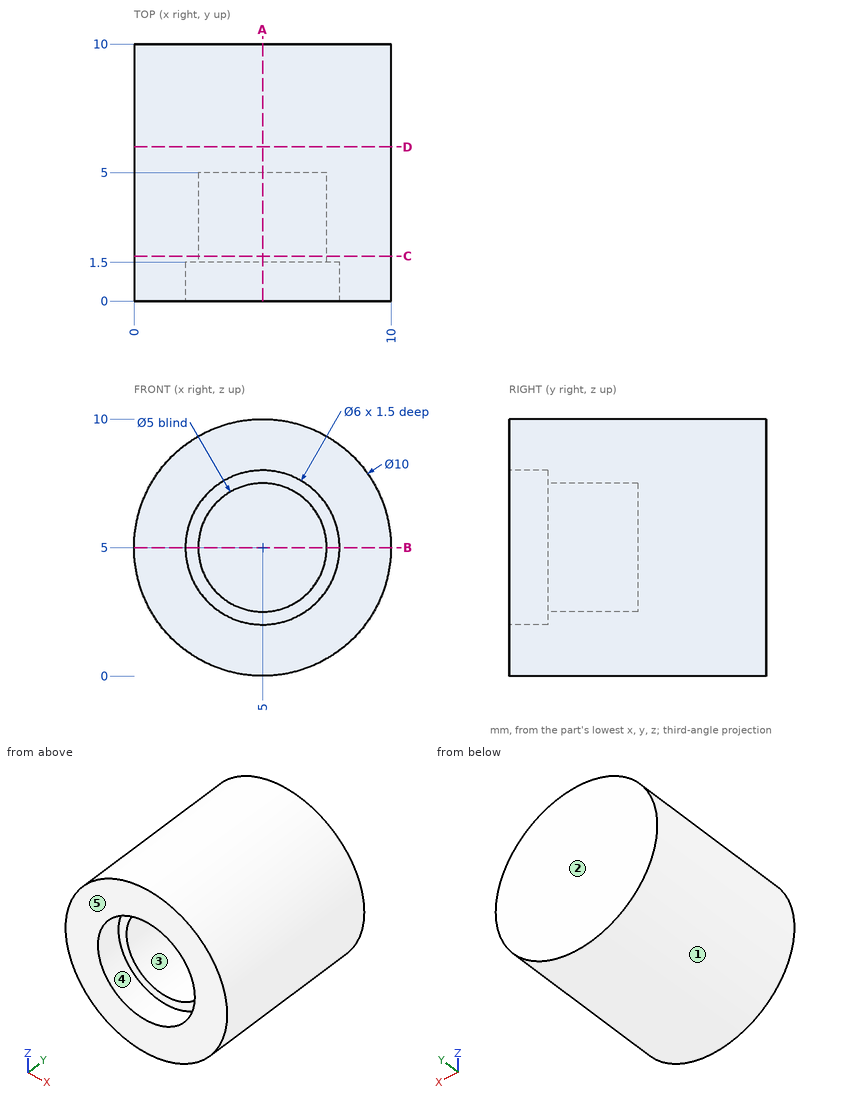
The figure shows three views and two pictorial views of one solid part (mm, origin at its lowest corner). Answer the questions. A direction names the side the tool comes from. Round coordinates to 2 decimals unless told otherwise and drop trailing zeros. Write each loop counter-clockwise with the first axis right and the second up, starting at its lowest first coordinate (ties: lowest second). Pieces come first, ordered by that corner, then holes. Notation, with made-up numbers: M -29.75,38.25 L 27.25,38.25 A29 ccw 27.25,76.25 Z; hole C -32,-15 d2. An arc over 180 degrees is marked long. Use a Markdown table: item, result.
1) The part is cut by section A-A (x = 5). Write down the section's boundary in (y, z).
Answers follow:
| item | result |
|---|---|
| outline | M 0,0 L 10,0 L 10,10 L 0,10 L 0,8 L 1.5,8 L 1.5,7.5 L 5,7.5 L 5,2.5 L 1.5,2.5 L 1.5,2 L 0,2 Z |
2) Straight lines are drawn through the part: line 1 along Z through (x, y) = (5, 2.95); line 2 along Y through (x, z) = (3.5, 6.5); line 3 along X through (y, z) = (4, 6.25). For each, find the intervals that lie inside material, in ascending order. Write a range as [from, to].
Answers follow:
| item | result |
|---|---|
| line 1 | z = [0, 2.5], [7.5, 10] |
| line 2 | y = [5, 10] |
| line 3 | x = [0.16, 2.83], [7.17, 9.84] |
3) The part is cut by section B-B (z = 5). Write down the section's boundary in (x, y).
Answers follow:
| item | result |
|---|---|
| outline | M 0,0 L 2,0 L 2,1.5 L 2.5,1.5 L 2.5,5 L 7.5,5 L 7.5,1.5 L 8,1.5 L 8,0 L 10,0 L 10,10 L 0,10 Z |
4) The part is cut by section C-C (y = 1.75). Write down the section's boundary in (x, z).
Answers follow:
| item | result |
|---|---|
| outline | C 5,5 d10; hole C 5,5 d5 |
5) Flat-ended cylindrical pins translate along their axes: pin 1 (4 mm diameter, centred on x = 2.5, y = 2, fed in from -Z); pin 2 (3 mm diameter, centred on x = 1.5, y = 5, fed in from +Z); pin 3 (1.5 mm diameter, centred on x = 1.5, y = 8.5, fed in from +Z). Find the tip coordinate at first contact, or state that the pin passes through.
Answers follow:
| item | result |
|---|---|
| pin 1 | stops at z = 0.03 |
| pin 2 | stops at z = 9.58 |
| pin 3 | stops at z = 9.18 |
6) For a pull along X with two mould halves and no side action, classify the marked faces 1, 2 and 3 as pulls with the +X half, pulls with the -X half, needs draft (parallel to the pull), parting line crosses it, or undercut.
Answers follow:
| item | result |
|---|---|
| face 1 | parting line crosses it |
| face 2 | needs draft |
| face 3 | undercut |
7) The part is cut by section D-D (y = 6). Write down the section's boundary in (x, z), plus the area to 3 significant figures.
Answers follow:
| item | result |
|---|---|
| outline | C 5,5 d10 |
| area | 78.5 mm2 |
8) A tool of negligible diameter and unlimited length cuts with its end or side. For the marked faces 4 and 5, from which of +Z, -Z, +X, -X, +Y, -Y can it reach the whole face along a straight path? Write none if from no direction.
Answers follow:
| item | result |
|---|---|
| face 4 | -Y |
| face 5 | +Z, -Z, +X, -X, -Y |
